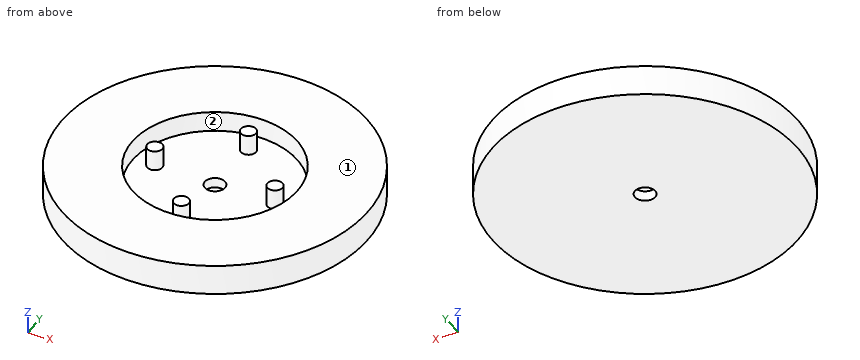
from build123d import *

# Parameters (mm, degrees)
SKETCH1_R           = 8.1
SKETCH1_R_2         = 0.75
SKETCH1_R_3         = 1
BOSS_EXTRUDE1_DEPTH = 1
SKETCH1_3_R         = 15
SKETCH1_3_R_2       = 8.1
SKETCH1_3_R_3       = 0.75
BOSS_EXTRUDE2_DEPTH = 3


with BuildPart() as part:
    # Sketch1 → Boss-Extrude1 (new body)
    # profile 1 of 5: a face of its own
    with BuildSketch(Plane.XY):
        Circle(SKETCH1_R)
        with Locations((0, 6)):
            Circle(SKETCH1_R_2, mode=Mode.SUBTRACT)
        with Locations((6, 0)):
            Circle(SKETCH1_R_2, mode=Mode.SUBTRACT)
        with Locations((0, -6)):
            Circle(SKETCH1_R_2, mode=Mode.SUBTRACT)
        with Locations((-6, 0)):
            Circle(SKETCH1_R_2, mode=Mode.SUBTRACT)
        Circle(SKETCH1_R_3, mode=Mode.SUBTRACT)
    # profile 2 of 5: a face of its own
    with BuildSketch(Plane.XY):
        with Locations((0, 6)):
            Circle(SKETCH1_R_2)
    # profile 3 of 5: a face of its own
    with BuildSketch(Plane.XY):
        with Locations((-6, 0)):
            Circle(SKETCH1_R_2)
    # profile 4 of 5: a face of its own
    with BuildSketch(Plane.XY):
        with Locations((6, 0)):
            Circle(SKETCH1_R_2)
    # profile 5 of 5: a face of its own
    with BuildSketch(Plane.XY):
        with Locations((0, -6)):
            Circle(SKETCH1_R_2)
    extrude(amount=BOSS_EXTRUDE1_DEPTH)

    # Sketch1_3 → Boss-Extrude2 (add)
    # profile 1 of 5: a face of its own
    with BuildSketch(Plane.XY):
        Circle(SKETCH1_3_R)
        Circle(SKETCH1_3_R_2, mode=Mode.SUBTRACT)
    # profile 2 of 5: a face of its own
    with BuildSketch(Plane.XY):
        with Locations((-6, 0)):
            Circle(SKETCH1_3_R_3)
    # profile 3 of 5: a face of its own
    with BuildSketch(Plane.XY):
        with Locations((0, 6)):
            Circle(SKETCH1_3_R_3)
    # profile 4 of 5: a face of its own
    with BuildSketch(Plane.XY):
        with Locations((6, 0)):
            Circle(SKETCH1_3_R_3)
    # profile 5 of 5: a face of its own
    with BuildSketch(Plane.XY):
        with Locations((0, -6)):
            Circle(SKETCH1_3_R_3)
    extrude(amount=BOSS_EXTRUDE2_DEPTH)


solid = part.part
Could you check a few things on this model? Use its own coordinates, in mm. Face numbers are marked on the shaded views. A direction names the side the tool comes from. Give positions to 0.01 mm unless a question says otherwise; leave off trailing zeros. Order: outer loops, then holes, each group sorted by start corner. A loop starts at its lowest first (then second) coordinate and runs counter-clockwise, first axis right, second up. Notation, with made-up numbers: (6.5, 61) - (53.5, 61) arc R19 cw to (53.5, 79) - close; hole circle Ø8 at (34.25, 23.25). An arc over 180 degrees is marked (long way). Return JSON: item names as keys, results as strings. Group by question number.
Q1. Suppose I cut it at C-C, the plane y = -7.5. Please give me the cut outline in (x, z).
Q2. Suppose I cut it at D-D, the plane x = 6. Please give me the cut outline in (y, z).
Q3. Suppose I cut it at B-B, the plane z = 0.4. Please give me the cut outline in (x, y).
Q4. Suppose I cut it at A-A, the plane x = 0. Please give me the cut outline in (y, z).
Q5. Will these pins go through, and if not, where does the flat tip stop? pin 1 Ø2 at (x, y) = (-3.5, -11) entering from -Z; pin 2 Ø1.6 at (x, y) = (0, 0) entering from -Z.
Q6. Please list where these lines run through material, in increasing order: line 1 along Y through (x, z) = (0, 1.6); line 2 along Y through (x, z) = (0, 0.6); line 3 along Y through (x, z) = (-6.5, 1.05). Write a range as [from, to].
Q7. Which directions (+Z, -Z, +X, -X, +Y, -Y) give clear straight access to the entire face, cutting with the end or side of a thin tool? Please do the marked faces 1 and 2.
Resolved:
{
 "1": {"outline": "(-12.99, 0) - (12.99, 0) - (12.99, 3) - (3.06, 3) - (3.06, 1) - (-3.06, 1) - (-3.06, 3) - (-12.99, 3) - close"},
 "2": {"outline": "(-13.75, 0) - (13.75, 0) - (13.75, 3) - (5.44, 3) - (5.44, 1) - (0.75, 1) - (0.75, 3) - (-0.75, 3) - (-0.75, 1) - (-5.44, 1) - (-5.44, 3) - (-13.75, 3) - close"},
 "3": {"outline": "circle Ø30 at (0, 0); hole circle Ø2 at (0, 0)"},
 "4": {"outline": "(-15, 0) - (-1, 0) - (-1, 1) - (-5.25, 1) - (-5.25, 3) - (-6.75, 3) - (-6.75, 1) - (-8.1, 1) - (-8.1, 3) - (-15, 3) - close; (1, 0) - (15, 0) - (15, 3) - (8.1, 3) - (8.1, 1) - (6.75, 1) - (6.75, 3) - (5.25, 3) - (5.25, 1) - (1, 1) - close"},
 "5": {"pin 1": "stops at z = 0", "pin 2": "passes through"},
 "6": {"line 1": "y = [-15, -8.1], [-6.75, -5.25], [5.25, 6.75], [8.1, 15]", "line 2": "y = [-15, -1], [1, 15]", "line 3": "y = [-13.52, -4.83], [-0.56, 0.56], [4.83, 13.52]"},
 "7": {"face 1": "+Z, +X, -X, +Y, -Y", "face 2": "+Z"}
}
